Design review of the part built by this model. Coordinates are the model's own, in mm. A direction names the side the tool comes from. Give positions to 0.01 mm unless a question says otherwise; leave off trailing zeros. Order: outer loops, then holes, each group sorted by start corner. A loop starts at its lowest first (then second) coordinate and runs counter-clockwise, first axis right, second up. Notation, with made-up numbers: M 12,6 L 62,6 A26 ccw 62,45 Z; hole C 18.25,8.5 d10. An arc over 180 degrees is marked long. Answer as a JSON object with one key per item and string values.
from build123d import *

# Parameters (mm, degrees)
SKETCH1_R           = 1
BOSS_EXTRUDE1_DEPTH = 3
SKETCH2_W           = 2.125
SKETCH2_H           = 16.25
CUT_EXTRUDE1_DEPTH  = 22.56965461
CUT_EXTRUDE2_DEPTH  = 3.5
FILLET1_R           = 0.333333333


with BuildPart() as part:
    # Sketch1 → Boss-Extrude1 (new, symmetric)
    with BuildSketch(Plane(origin=(0, 0, 0), x_dir=(0, 0, -1), z_dir=(1, 0, 0))):
        with BuildLine():
            Line((2.75, 0), (2.75, 15))
            Line((2.75, 15), (3.75, 15))
            Line((3.75, 15), (3.75, 16))
            Line((3.75, 16), (6.25, 16))
            Line((6.25, 16), (6.75, 16.5))
            Line((6.75, 16.5), (6.75, 18))
            Line((6.75, 18), (5.15, 18))
            Line((5.15, 18), (5.15, 17.75))
            Line((5.15, 17.75), (3.55, 17.75))
            Line((3.55, 17.75), (3.55, 17.5))
            Line((3.55, 17.5), (1.95, 17.5))
            Line((1.95, 17.5), (1.95, 17.25))
            Line((1.95, 17.25), (0.35, 17.25))
            Line((0.35, 17.25), (0.35, 17))
            Line((0.35, 17), (-4.75, 17))
            Line((-4.75, 17), (-4.75, 13.5))
            Line((-4.75, 13.5), (-2.75, 13.5))
            Line((-2.75, 13.5), (-2.75, 0))
            ThreePointArc((-2.75, 0), (0, -2.75), (2.75, 0))
        make_face()
        Circle(SKETCH1_R, mode=Mode.SUBTRACT)
    extrude(amount=BOSS_EXTRUDE1_DEPTH, both=True)

    # Sketch2 → Cut-Extrude1 (cut, through all)
    with BuildSketch(Plane.XY.offset(4.75)):
        with Locations((1.9375, 5.375)):
            Rectangle(SKETCH2_W, SKETCH2_H)
        with Locations((-1.9375, 5.375)):
            Rectangle(SKETCH2_W, SKETCH2_H)
    extrude(amount=-CUT_EXTRUDE1_DEPTH, mode=Mode.SUBTRACT)

    # Sketch3 → Cut-Extrude2 (cut)
    with BuildSketch(Plane(origin=(0, 17, 0), x_dir=(1, 0, 0), z_dir=(0, 1, 0))):
        Polygon((-0.875, -4.25), (0.875, -4.25), (1.375, -4.75), (-1.375, -4.75), align=None)
    extrude(amount=-CUT_EXTRUDE2_DEPTH, mode=Mode.SUBTRACT)

    # Fillet1
    fillet1_edges = [part.edges().sort_by_distance(p)[0] for p in [
        (-2.1875, 17, 4.75),
        (2.1875, 17, 4.75),
    ]]
    fillet(fillet1_edges, radius=FILLET1_R)


solid = part.part
(1) We need section C-C (y = 16.25). Write out the cut boundary in (x, z) (3 decimals).
Checked values:
{"outline": "M -3,-6.5 L 3,-6.5 L 3,4.75 L 1.375,4.75 L 0.875,4.25 L -0.875,4.25 L -1.375,4.75 L -3,4.75 Z"}
(2) We need section A-A (z = 0). Write out the cut boundary in (x, y) (3 decimals).
Checked values:
{"outline": "M -3,13.5 L -0.875,13.5 L -0.875,1 L 0.875,1 L 0.875,13.5 L 3,13.5 L 3,17 L -3,17 Z; M -0.875,-2.75 L 0.875,-2.75 L 0.875,-1 L -0.875,-1 Z"}
(3) To check wall thickness, follow L1, parallel to Z at x = 0.3, y = 0; L2, parallel to Y at x = 0.1, z = 0; L3, parallel to X at y = 8.5, z = -1 (3 decimals). State the ranges of each line that lie inside material, in increasing order. Write a range as from..to.
Checked values:
{"L1": "z = -2.75..-1, 1..2.75", "L2": "y = -2.75..-1, 1..17", "L3": "x = -0.875..0.875"}
(4) We need section D-D (z = 2). Write out the cut boundary in (x, y) (3 decimals), plus the area to 3 significant figures.
Checked values:
{"outline": "M -3,13.5 L -0.875,13.5 L -0.875,-1.887 L 0.875,-1.887 L 0.875,13.5 L 3,13.5 L 3,17 L -3,17 Z", "area": "47.9 mm^2"}
(5) Insertion check: pin 1 (3 mm diameter, centred on y = 4, z = 1, fed in from -X) (3 decimals); pin 2 (4.5 mm diameter, centred on y = 5, z = 0, fed in from +X) (3 decimals); pin 3 (0.5 mm diameter, centred on x = 1.5, z = -1, fed in from +Y). Each pin has a flat end and moves straight along its axis. Give the tip position at first contact, or say it passes through.
Checked values:
{"pin 1": "stops at x = -0.875", "pin 2": "stops at x = 0.875", "pin 3": "stops at y = 17.25"}
(6) Tool access review of faces 1 (the flat face through (3, 16, -1)), 2 (the flat face through (-0.875, 5, 0)), 3 (the flat face through (0, 17, 2)), 4 (the flat face through (0, 7, 2.75)), 5 (the flat face through (0, 15.5, -3.75)): name each direction out of +Z, -Z, +X, -X, +Y, -Y from which nothing blocks a thin tool from reaching the whole face with its end or side.
Checked values:
{"face 1": "+Z, -Z, +X, +Y, -Y", "face 2": "+Z, -Z, -X, -Y", "face 3": "+Z, +X, -X, +Y", "face 4": "+Z, +X, -X, -Y", "face 5": "-Z, +X, -X, -Y"}
(7) Draft analysis for pull direction X (two halves, no side actions). For faces 6 (the flat face through (0, 18, -6)), 7 (the flat face through (-3, 16, -1)), 8 (the flat face through (0, 15, 4.25)), 9 (the flat face through (0.875, 5, 0)), state which applies: +X half, -X half, draft (parallel to the pull), parting line (faces both ways), or undercut.
Checked values:
{"face 6": "draft", "face 7": "-X half", "face 8": "undercut", "face 9": "+X half"}
(8) We need section B-B (x = 0.45). Write out the cut boundary in (y, z), plus the area to 3 significant figures.
Checked values:
{"outline": "M 0,-2.75 L 15,-2.75 L 15,-3.75 L 16,-3.75 L 16,-6.25 L 16.5,-6.75 L 18,-6.75 L 18,-5.15 L 17.75,-5.15 L 17.75,-3.55 L 17.5,-3.55 L 17.5,-1.95 L 17.25,-1.95 L 17.25,-0.35 L 17,-0.35 L 17,4.25 L 13.5,4.25 L 13.5,2.75 L 0,2.75 A2.75 ccw Z; hole C 0,0 d2", "area": "116 mm^2"}
